For this review, take the finished solid that the model builds, in its own axes (mm). A direction names the side the tool comes from. Coordinates: 2 decimals unless noted, no trailing zeros. Loops run counter-clockwise (first coordinate to the right, second up) from the corner with the lowest first, then second, coordinate; pieces in that order, holes last. Notation, with made-up numbers: M -23,47 L 10,47 A21 ccw 10,70 Z; hole C 17.25,71.25 d4. An arc over 180 degrees is marked long. Put each result on its own line as item: value.
```python
from build123d import *

# Parameters (mm, degrees)
F1_DEPTH = 2
F3_DEPTH = 4
F5_DEPTH = 25
F6_R     = 4.99999
F8_DEPTH = 1


# Not quite as in the source:
# - a fillet or chamfer is up to 0.001 mm smaller than in the source, because OpenCascade refuses the exact size


with BuildPart() as f1:
    # F0 (on Front) → F1 (new body)
    with BuildSketch(Plane.XZ):
        Polygon((-50, 2.2), (-50, 0), (-14.6446609407, -35.3553390593), (-0.5025253169, -21.2132034356), (-7.5735931288, -14.1421356237), (14.1421356237, 7.5735931288), (21.2132034356, 0.5025253169), (35.3553390593, 14.6446609407), (0, 50), (-2.2, 50), (-2.2, 2.2), align=None)
        Polygon((-32.3101722444, 41.9320036632), (-50, 2.2), (-2.2, 2.2), (-2.2, 50), align=None)
    extrude(amount=F1_DEPTH)

    # F2 (on face) → F3 (join)
    with BuildSketch(Plane(origin=(0, 0, 0), x_dir=(-1, 0, 0), z_dir=(0, 1, 0))):
        Polygon((0, 0), (0, 50), (-2, 48), (-2, -2), (48, -2), (50, 0), align=None)
        Polygon((4.2, 45.3229968935), (2.2, 45.8588952784), (2.2, 2.2), (45.621454886, 2.2), (44.7309975154, 4.2), (4.2, 4.2), align=None)
    extrude(amount=F3_DEPTH)

    # F4 (on face) → F5 (cut)
    with BuildSketch(Plane(origin=(0, 0, 0), x_dir=(-1, 0, 0), z_dir=(0, 1, 0))):
        Polygon((7.5735934344, -21.2132034356), (14.6446609407, -28.2842709419), (35.9289316665, -7.0000002161), (7.5025258386, -7.0000002161), (14.6446612462, -14.1421356237), align=None)
        Polygon((-14.1421356237, 14.6446612462), (-7.0000002161, 7.5025258386), (-7.0000002161, 35.9289316665), (-28.2842709419, 14.6446609407), (-21.2132034356, 7.5735934344), align=None)
    extrude(amount=-F5_DEPTH, mode=Mode.SUBTRACT)

    # F6 (radius 5 in the source; OpenCascade refuses exactly that, so slightly less here)
    f6_edges = [f1.edges().sort_by_distance(p)[0] for p in [
        (35.355339, -1, 14.644661),
        (21.213203, -1, 0.502525),
        (-14.644661, -1, -35.355339),
        (-0.502525, -1, -21.213203),
        (-14.644661, -1, -14.142136),
        (14.142136, -1, 14.644661),
        (14.142136, -1, 7.573593),
        (21.213203, -1, 7.573593),
        (28.284271, -1, 14.644661),
        (-14.644661, -1, -28.284271),
        (-7.573593, -1, -21.213203),
    ]]
    fillet(f6_edges, radius=F6_R)

    # F7 (on face) → F8 (cut)
    with BuildSketch(Plane(origin=(0, 0, 0), x_dir=(-1, 0, 0), z_dir=(0, 1, 0))):
        Polygon((2.2, 50), (0, 50), (0, 0), (50, 0), (50, 2.2), (45.621454886, 2.2), (2.2, 2.2), (2.2, 45.8588952784), align=None)
    extrude(amount=-F8_DEPTH, mode=Mode.SUBTRACT)


solid = f1.part
```
(1) Draft analysis for pull direction Z (two halves, no side actions). For faces 4 (the flat face through (-14, -1, 1)), 5 (the flat face through (15.75, -0.99, 27.18)), 6 (the cylindrical face through (-14.7, -1.014, -33.284)), 7 (the flat face through (-9, -2, 9)), state which applies: +Z half, -Z half, draft (parallel to the pull), parting line (faces both ways), or undercut.
Determined:
face 4: undercut
face 5: undercut
face 6: -Z half
face 7: draft
(2) For pin 1 (1.5 mm diameter, centred on x = -28, y = 1.5, fed in from +Z); pin 2 (2 mm diameter, centred on y = 3, z = 20, fed in from -X); pin 3 (25 mm diameter, centred on x = -35.5, z = 31.5, fed in from +Y); pin 4 (1 mm diameter, centred on y = 1.5, z = -7.5, fed in from +X), all flat-tipped, find the tip position at first contact; note any pin that passes through.
Determined:
pin 1: stops at z = 4.2
pin 2: stops at x = -4.2
pin 3: stops at y = 0
pin 4: passes through
(3) Tool access review of faces 1 (the cylindrical face through (26.213, -1.014, 14.59)), 2 (the flat face through (-3.21, 1.97, 45.59)), 3 (the flat face through (0, 2, 25)): name each direction out of +Z, -Z, +X, -X, +Y, -Y from which nothing blocks a thin tool from reaching the whole face with its end or side.
Determined:
face 1: +Y, -Y
face 2: +Z, -X, +Y
face 3: +Z, +Y
(4) Wall thickness on line 1 along Z through (x, y) = (-44.5, 2.5); line 2 along X through (y, z) = (1.15, 41.5); line 3 along X through (y, z) = (-0.2, 32): over which ranges is each line inside the solid? List them lowest first. Write a range as [from, to].
Determined:
line 1: z = [-2, 0], [2.2, 4.2]
line 2: x = [-4.2, -2.2], [0, 2]
line 3: x = [-36.73, -2.2], [0, 7], [10.93, 18]
(5) Add section A-A (y = 1.75). Write out the cut boundary in (x, z).
Determined:
outline: M -50,0 L -48,-2 L 2,-2 L 2,48 L 0,50 L 0,0 Z; M -45.62,2.2 L -2.2,2.2 L -2.2,45.86 L -4.2,45.32 L -4.2,4.2 L -44.73,4.2 Z
(6) Add section D-D (x = -40.5). Write out the cut boundary in (y, z).
Determined:
outline: M -2,-9.5 L 0,-9.5 L 0,-2 L 4,-2 L 4,0 L -1,0 L -1,2.2 L 4,2.2 L 4,4.2 L 0,4.2 L 0,23.54 L -2,23.54 Z
(7) Add section B-B (x = -14). Write out the cut boundary in (y, z), plus the area to 3 significant figures.
Determined:
outline: M -2,-33.24 L 0,-33.24 L 0,-26.17 L -2,-26.17 Z; M -2,-7 L 0,-7 L 0,-2 L 4,-2 L 4,0 L -1,0 L -1,2.2 L 4,2.2 L 4,4.2 L 0,4.2 L 0,46.84 L -2,46.84 Z
area: 136 mm^2
(8) Add section C-C (z = 30). Write out the cut boundary in (x, y), plus the area to 3 significant figures.
Determined:
outline: M -37.62,-2 L 7,-2 L 7,0 L 2,0 L 2,4 L 0,4 L 0,-1 L -2.2,-1 L -2.2,4 L -4.2,4 L -4.2,0 L -37.62,0 Z; M 12.93,-2 L 20,-2 L 20,0 L 12.93,0 Z
area: 117 mm^2
